Check sheet for the modelled part. Datum: model origin and axes. Units: mm. A direction names the side the tool comes from. Round coordinates to 2 decimals unless told otherwise and drop trailing zeros. Loops run counter-clockwise (first coordinate to the right, second up) from the corner with the lowest first, then second, coordinate; pieces in that order, holes last. Notation, with made-up numbers: (-2.75, 74) - (24.25, 74) arc R15 ccw to (24.25, 98) - close; hole circle Ø7 at (-12, 60). An arc over 180 degrees is marked (long way). Return JSON: item names as keys, results as strings.
from build123d import *

# Parameters (mm, degrees)
F0_R     = 12
F1_DEPTH = 105.7
F3_DEPTH = 105.7
F4_W     = 84
F4_H     = 98.5
F5_DEPTH = 40
F6_R     = 21.461704
F7_DEPTH = 20


with BuildPart() as f1:
    # F0 (on Front) → F1 (new body)
    with BuildSketch(Plane.XZ):
        with BuildLine():
            Line((90, 22.5), (0, 22.5))
            Line((0, 22.5), (-64.5, 22.5))
            ThreePointArc((-64.5, 22.5), (-87, 0), (-64.5, -22.5))
            Line((-64.5, -22.5), (0, -22.5))
            Line((0, -22.5), (90, -22.5))
            ThreePointArc((90, -22.5), (112.5, 0), (90, 22.5))
        make_face()
        with Locations((90, 0)):
            Circle(F0_R, mode=Mode.SUBTRACT)
    extrude(amount=F1_DEPTH)

    # F2 (on face) → F3 (join)
    with BuildSketch(Plane.XZ.offset(105.7)):
        Polygon((-84.272794, -1.934636), (-87, 0), (-87, -22.5), (-64.5, -22.5), (-70.418127, -18.801184), (-80.156557, -10.970287), align=None)
    extrude(amount=-F3_DEPTH)

    # F4 (on face) → F5 (cut)
    with BuildSketch(Plane.XY.offset(22.5)):
        with Locations((0, -55.45)):
            Rectangle(F4_W, F4_H)
    extrude(amount=-F5_DEPTH, mode=Mode.SUBTRACT)

    # F6 (on face) → F7 (join)
    with BuildSketch(Plane.XZ.offset(105.7)):
        with Locations((90, 0)):
            Circle(F6_R)
    extrude(amount=F7_DEPTH)


solid = f1.part
Q1. Tool access check on faces 1 (the face through (90, -125.7, 0)), 2 (the face through (78.01, -52.11, 0.53)), 3 (the face through (0, -52, -22.5)), 4 (the face through (42, -56, 3)), 5 (the face through (68.56, -115.56, 0.94)). Record the directions out of +Z, -Z, +X, -X, +Y, -Y that give a thin tool (end or side, any length) a straight path to the whole face; none if there is none.
Answer key:
{"face 1": "+Z, -Z, +X, -X, -Y", "face 2": "+Y", "face 3": "-Z, +X, -X, +Y, -Y", "face 4": "+Z", "face 5": "-Y"}
Q2. Sectioned sample at B-B (z = -5.5). Enter the section's corners in (x, y) (3 decimals).
Answer key:
{"outline": "(-87, -105.7) - (69.255, -105.7) - (69.255, -125.7) - (110.745, -125.7) - (110.745, -105.7) - (111.817, -105.7) - (111.817, 0) - (100.665, 0) - (100.665, -105.7) - (79.335, -105.7) - (79.335, 0) - (-87, 0) - close; hole (-42, -104.7) - (42, -104.7) - (42, -6.2) - (-42, -6.2) - close"}
Q3. Scan lines: probe 1 along Z at (x, y) = (90, -57); probe 2 along Y at (x, z) = (16.5, 15); probe 3 along X at (y, z) = (-95, -10.5). Record each from-to range of solid material in increasing order. Write a range as [from, to].
Answer key:
{"probe 1": "z = [-22.5, -12], [12, 22.5]", "probe 2": "y = [-105.7, -104.7], [-6.2, 0]", "probe 3": "x = [-87, -42], [42, 84.19], [95.81, 109.9]"}
Q4. Sectioned sample at C-C (x = 56). Enter the section's corners in (y, z).
Answer key:
{"outline": "(-105.7, -22.5) - (0, -22.5) - (0, 22.5) - (-105.7, 22.5) - close"}
Q5. Depth check by flat-ended pin: P1, Ø8, axis at y = -78, z = 9.5, coming from the +X side; P2, Ø20, axis at x = 6, z = -0.5, coming from the -Y side; P3, Ø4, axis at y = -75.5, z = 12.5, coming from the +X side. Enter the tip coordinate at first touch or a pass-through.
Answer key:
{"P1": "stops at x = 111.82", "P2": "stops at y = -105.7", "P3": "stops at x = 109.9"}
Q6. Sectioned sample at A-A (y = -13). Enter the section's corners in (x, z).
Answer key:
{"outline": "(-87, -22.5) - (90, -22.5) arc R22.5 ccw to (90, 22.5) - (42, 22.5) - (42, -17.5) - (-42, -17.5) - (-42, 22.5) - (-64.5, 22.5) arc R22.5 ccw to (-87, 0) - close; hole circle Ø24 at (90, 0)"}
Q7. Draft check along Y on faces 6 (the face through (11, 0, 0)), 7 (the face through (-1, -6.2, 3)), 8 (the face through (-80.234, -52.11, 16.084)). Enter one of: released by +Y, released by -Y, zero draft, split by the parting line, or undercut.
Answer key:
{"face 6": "released by +Y", "face 7": "undercut", "face 8": "zero draft"}
